Autodesk Inventor part; units mm, degrees
ref_plane "YZ Plane" through (0, 0, 0) normal (1, 0, 0) x (0, 1, 0)
ref_plane "XZ Plane" through (0, 0, 0) normal (0, 1, 0) x (-1, 0, 0)
ref_plane "XY Plane" through (0, 0, 0) normal (0, 0, 1) x (1, 0, 0)
sketch "스케치1" plane through (0, 0, 0) normal (1, 0, 0) x (0, 1, 0)
  line L0 (-7.5, 10) -> (7.5, 10)
  line L1 (7.5, 10) -> (7.5, -10)
  line L2 (7.5, -10) -> (-7.5, -10)
  line L3 (-7.5, -10) -> (-7.5, 10)
  line L4 (-7.5, 10) -> (7.5, -10) construction
  line L5 (7.5, 10) -> (-7.5, -10) construction
  circle A0 centre (0, 0) radius 1.25
  line L6 (7.5, 10) -> (7.5, -10)
  line L7 (7.5, -10) -> (10.5, -10)
  line L8 (10.5, -10) -> (10.5, 10)
  line L9 (10.5, 10) -> (7.5, 10)
  line L10 (10.5, -6) -> (7.5, -6)
  line L11 (10.5, 6) -> (7.5, 6)
  dimension "d0" = 15
  dimension "d1" = 20
  dimension "d2" = 2.5
  dimension "d5" = 3
  dimension "d6" = 6
  dimension "d7" = 6
extrude "돌출1" add sketch "스케치1" along normal blind 3 contours L0 L1 L2 L3
extrude "돌출2" add sketch "스케치1" along normal blind 12.5 contours L11 L8 L10 L1
chamfer "모따기1" distance 3 angle 45 2 edges at (1.5, 7.5, 6) (1.5, 7.5, -6)
properties part number "latch"
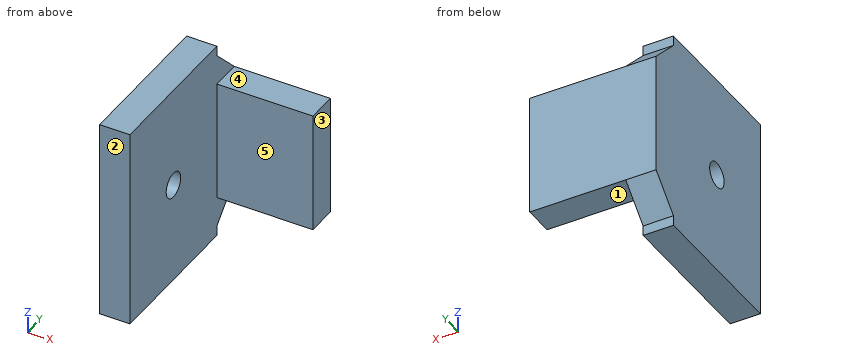
The model under review builds one solid part; all positions refer to its coordinate system, in mm. Face numbers are marked on the shaded views. A direction names the side the tool comes from. Round coordinates to 2 decimals unless told otherwise and drop trailing zeros. Write each loop counter-clockwise with the first axis right and the second up, starting at its lowest first coordinate (ties: lowest second). Pieces come first, ordered by that corner, then holes.
(1) Insertion check: pin 1 (1.5 mm diameter, centred on y = 0, z = 0, fed in from -X); pin 2 (1 mm diameter, centred on y = -4, z = -4, fed in from +X); pin 3 (1 mm diameter, centred on x = 7.5, z = -3.5, fed in from -Y); pin 4 (0.8 mm diameter, centred on x = 1.5, z = -9.5, fed in from +Y). Each pin has a flat end and moves straight along its axis. Give the tip position at first contact, or say it passes through.
(2) Machinability: for the marked faces 1, 2, 3, 4 and 5, which of the approach directions +Z, -Z, +X, -X, +Y, -Y give a long, thin tool a straight path to every point of the face, cutting with its end or side? Answer none if there is none.
(3) We need section D-D on x = 8. Give the boundary of the cut face in (y, z), and give its area (3 significant figures).
(4) We need section C-C on z = 0. Give the boundary of the cut face in (x, y), and give its area (3 significant figures).
(5) Wall thickness on L1, parallel to Z at x = 0.8, y = 0; L2, parallel to Y at x = 4.5, z = 1.5; L3, parallel to X at y = 0.5, z = 7.25: over which ranges is each line inside the solid? List them lowest first.
(6) We need section A-A on y = 0.75. Give the boundary of the cut face in (x, z), and give its area (3 significant figures).
Findings below:
1. pin 1: passes through
1. pin 2: stops at x = 3
1. pin 3: stops at y = 7.5
1. pin 4: stops at y = 7.5
2. face 1: -Z, +X, +Y, -Y
2. face 2: +Z, -Z, +X, -X, -Y
2. face 3: +Z, -Z, +X, +Y, -Y
2. face 4: +Z, +X, +Y, -Y
2. face 5: +Z, -Z, +X, -Y
3. outline: (7.5, -6) - (10.5, -6) - (10.5, 6) - (7.5, 6) - close
3. area: 36.0 mm2
4. outline: (0, -7.5) - (3, -7.5) - (3, -1.25) - (0, -1.25) - close; (0, 1.25) - (3, 1.25) - (3, 7.5) - (12.5, 7.5) - (12.5, 10.5) - (0, 10.5) - close
4. area: 75.0 mm2
5. L1: z = -10 to -1.25, 1.25 to 10
5. L2: y = 7.5 to 10.5
5. L3: x = 0 to 3
6. outline: (0, -10) - (3, -10) - (3, -1) - (0, -1) - close; (0, 1) - (3, 1) - (3, 10) - (0, 10) - close
6. area: 54.0 mm2
